```python
from build123d import *

# Parameters (mm, degrees)
CHAMFER_1_SIZE = 0.5
CHAMFER_2_SIZE = 0.2


with BuildPart() as part:
    # Эскиз1 → Повернуть1 (revolve)
    with BuildSketch(Plane.XY, mode=Mode.PRIVATE) as revolve_1_sk:
        with BuildLine():
            Line((0.833368845, 16.5), (3.5, 16.5))
            Line((3.5, 16.5), (3.5, 18.5))
            Line((3.5, 18.5), (-3.5, 18.5))
            Line((-3.5, 18.5), (-3.5, 16.5))
            Line((-3.5, 16.5), (-0.833368845, 16.5))
            ThreePointArc((-0.833368845, 16.5), (-0.47911964, 16.67422796), (-0.091683865, 16.75))
            Line((-0.091683865, 16.75), (0.091683865, 16.75))
            ThreePointArc((0.091683865, 16.75), (0.47911964, 16.67422796), (0.833368845, 16.5))
        make_face()
    revolve(revolve_1_sk.sketch.rotate(Axis((0, 0, 0), (1, 0, 0)), 90), axis=Axis((0, 0, 0), (1, 0, 0)))

    # Фаска1
    chamfer_1_edges = [part.edges().sort_by_distance(p)[0] for p in [
        (-3.5, 0, -18.5),
        (3.5, 0, -18.5),
    ]]
    chamfer(chamfer_1_edges, length=CHAMFER_1_SIZE)

    # Фаска2
    chamfer_2_edges = [part.edges().sort_by_distance(p)[0] for p in [
        (3.5, 0, -16.5),
        (-3.5, 0, -16.5),
    ]]
    chamfer(chamfer_2_edges, length=CHAMFER_2_SIZE)


solid = part.part
```
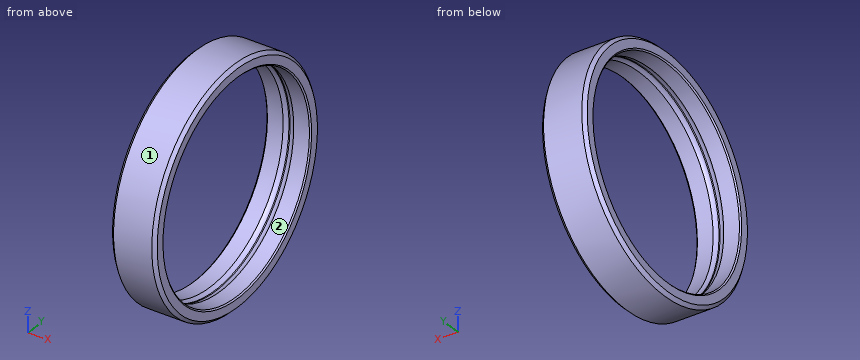
Geometry check sheet. Reference: the model listing, model coordinates, mm. Face numbers are marked on the shaded views. Give positions to 0.01 mm unless a question says otherwise; leave off trailing zeros. Order: outer loops, then holes, each group sorted by start corner. A loop starts at its lowest first (then second) coordinate and runs counter-clockwise, first axis right, second up.
1. Release check for a two-part mould opening along Z. For the marked faces 1 and 2 record: pulls with the +Z half, pulls with the -Z half, needs draft (parallel to the pull), parting line crosses it, or undercut.
2. Section check C-C, the plane x = -1.5. Enter the section's corners in (y, z).
3. Gauge pin test, flat ends, axial feed: pin 1 Ø2 at (x, z) = (-1.5, -9.5) entering from -Y; pin 2 Ø1 at (x, z) = (2, 9.5) entering from -Y; pin 3 Ø10 at (y, z) = (12.5, -8) entering from +X; pin 4 Ø4 at (x, z) = (-2.5, -3.5) entering from +Y. Record the tip position at first contact, or that the pin passes through.
4. Thickness scan on L1, parallel to Y at x = -1.4, z = 0; L2, parallel to Y at x = 0, z = 0; L3, parallel to Z at x = -3, y = -4. Record the ranges inside material, lowest first.
5. Section check A-A, the plane y = 0. Enter the section's corners in (x, z).
Values follow:
1. face 1: parting line crosses it
1. face 2: undercut
2. outline: circle Ø37 at (0, 0); hole circle Ø33 at (0, 0)
3. pin 1: stops at y = -16.43
3. pin 2: stops at y = -16.16
3. pin 3: stops at x = 3.5
3. pin 4: stops at y = 18.44
4. L1: y = -18.5 to -16.5, 16.5 to 18.5
4. L2: y = -18.5 to -16.75, 16.75 to 18.5
4. L3: z = -18.06 to -16.01, 16.01 to 18.06
5. outline: (-3.5, -18) - (-3, -18.5) - (3, -18.5) - (3.5, -18) - (3.5, -16.7) - (3.3, -16.5) - (0.83, -16.5) arc R1.5 cw to (0.09, -16.75) - (-0.09, -16.75) arc R1.5 cw to (-0.83, -16.5) - (-3.3, -16.5) - (-3.5, -16.7) - close; (-3.5, 16.7) - (-3.3, 16.5) - (-0.83, 16.5) arc R1.5 cw to (-0.09, 16.75) - (0.09, 16.75) arc R1.5 cw to (0.83, 16.5) - (3.3, 16.5) - (3.5, 16.7) - (3.5, 18) - (3, 18.5) - (-3, 18.5) - (-3.5, 18) - close
